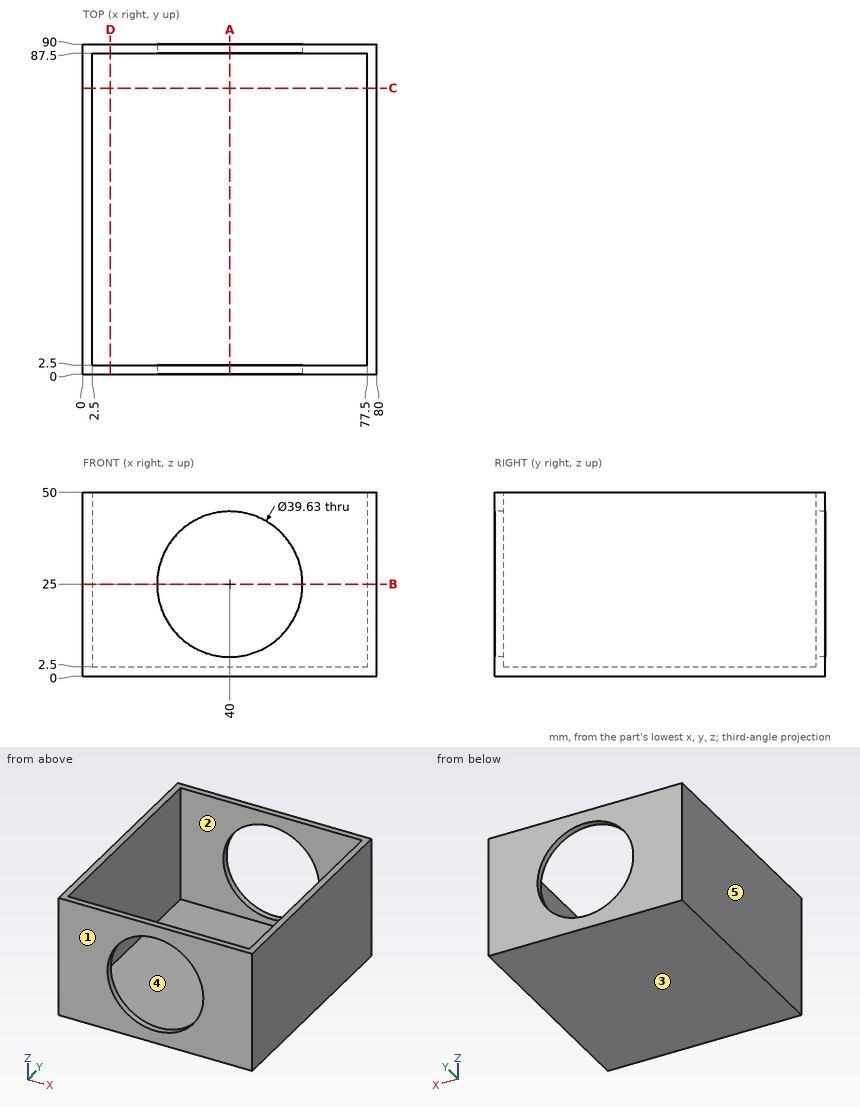
Job drawing, mm, ordinate dimensions from the low corner. One solid piece. A direction names the side the tool comes from. Coordinates: 2 decimals unless noted, no trailing zeros. Order: outer loops, then holes, each group sorted by start corner. A loop starts at its lowest first (then second) coordinate and runs counter-clockwise, first axis right, second up. Notation, with made-up numbers: (62.5, 33.25) -> (85.5, 33.25) arc R18 ccw to (85.5, 61.25) -> close; hole circle Ø1 at (-25, 54). An arc over 180 degrees is marked (long way). Put each result on its own line as item: value. Start each with the question number.
(1) Band-saw the part on A-A (x = 40). Give the cut face in (y, z) (3 decimals), then the cut area to 3 significant figures.
(2) Mould opens along X. For the marked faces 3, 4 and 5 say: pulls with the +X half, pulls with the -X half, needs draft (parallel to the pull), parting line crosses it, or undercut.
(3) Probe line 1 along X through (y, z) = (72, 15); line 2 along Z through (x, y) = (40, 1) (3 decimals); line 3 along Y through (x, z) = (16, 32). List the from-to ranges inside material, lowest first. Write a range as [from, to].
(4) Pin check, flat tips, straight feed: pin 1 Ø6 at (x, z) = (55, 23.5) entering from -Y; pin 2 Ø10 at (x, y) = (50, 19) entering from +Z. Stop position of each tip, or through.
(5) Band-saw the part on C-C (y = 78). Give the cut face in (x, z), then the cut area to 4 significant figures.
(6) Band-saw the part on B-B (z = 25). Give the cut face in (x, y) (3 decimals), then the cut area to 3 significant figures.
(7) Band-saw the part on D-D (x = 7.5). Give the cut face in (y, z).
(8) Which spindle directions (+Z, -Z, +X, -X, +Y, -Y) get a long thin tool onto all of the face, cutting with end or side? Do the marked faces 1 and 2. Say none if no direction does.
Determined:
1. outline: (0, 0) -> (90, 0) -> (90, 5.185) -> (87.5, 5.185) -> (87.5, 2.5) -> (2.5, 2.5) -> (2.5, 5.185) -> (0, 5.185) -> close; (0, 44.815) -> (2.5, 44.815) -> (2.5, 50) -> (0, 50) -> close; (87.5, 44.815) -> (90, 44.815) -> (90, 50) -> (87.5, 50) -> close
1. area: 264 mm²
2. face 3: needs draft
2. face 4: undercut
2. face 5: pulls with the -X half
3. line 1: x = [0, 2.5], [77.5, 80]
3. line 2: z = [0, 5.185], [44.815, 50]
3. line 3: y = [0, 2.5], [87.5, 90]
4. pin 1: passes through
4. pin 2: stops at z = 2.5
5. outline: (0, 0) -> (80, 0) -> (80, 50) -> (77.5, 50) -> (77.5, 2.5) -> (2.5, 2.5) -> (2.5, 50) -> (0, 50) -> close
5. area: 437.5 mm²
6. outline: (0, 0) -> (20.185, 0) -> (20.185, 2.5) -> (2.5, 2.5) -> (2.5, 87.5) -> (20.185, 87.5) -> (20.185, 90) -> (0, 90) -> close; (59.815, 0) -> (80, 0) -> (80, 90) -> (59.815, 90) -> (59.815, 87.5) -> (77.5, 87.5) -> (77.5, 2.5) -> (59.815, 2.5) -> close
6. area: 627 mm²
7. outline: (0, 0) -> (90, 0) -> (90, 50) -> (87.5, 50) -> (87.5, 2.5) -> (2.5, 2.5) -> (2.5, 50) -> (0, 50) -> close
8. face 1: +Z, -Z, +X, -X, -Y
8. face 2: +Z
